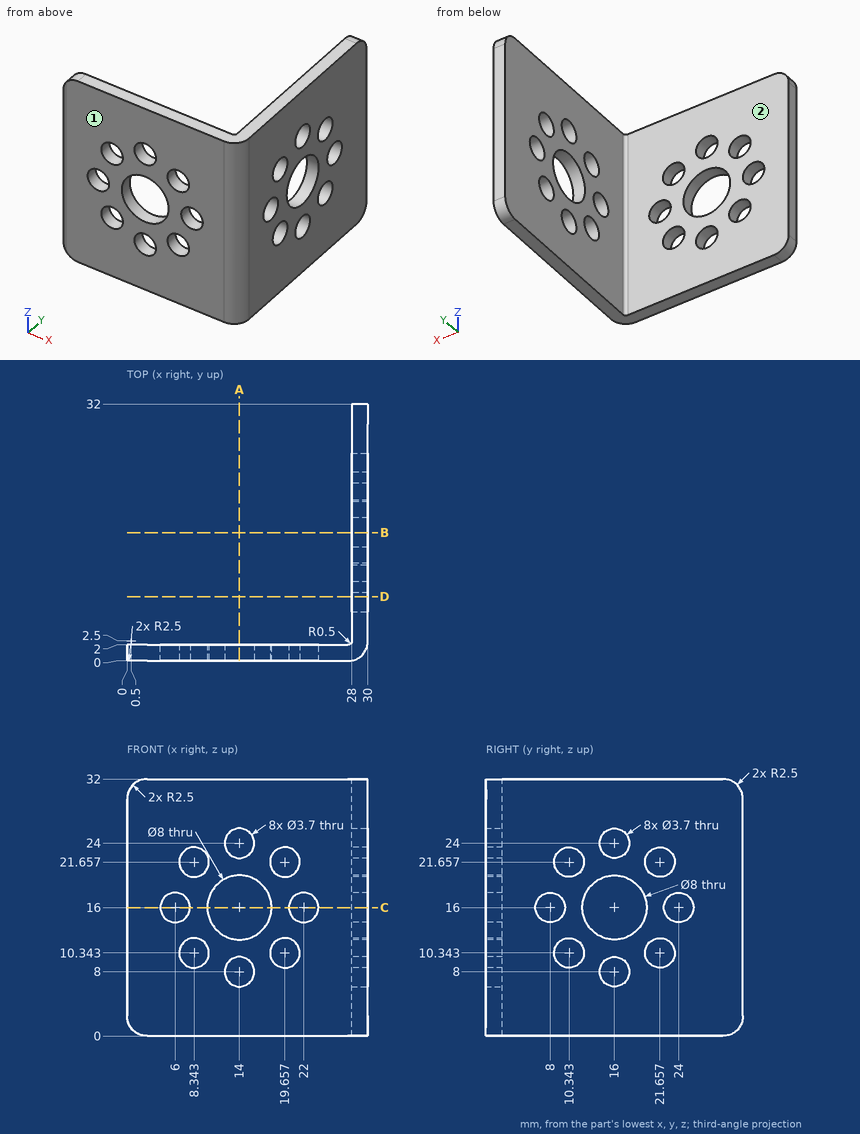
Answer from the drawing. Dimensions are ordinates in mm from the lowest x, y and z of the part. A direction names the side the tool comes from. Round coordinates to 2 decimals unless told otherwise and drop trailing zeros. Loops run counter-clockwise (first coordinate to the right, second up) from the corner with the lowest first, then second, coordinate; pieces in that order, holes last.
(1) The part is cut by section D-D, the plane y = 8. Give the vertices of the cut face in (x, z), and give its area (3 significant figures).
Computed values:
outline: (28, 0) - (30, 0) - (30, 14.15) - (28, 14.15) - close; (28, 17.85) - (30, 17.85) - (30, 32) - (28, 32) - close
area: 56.6 mm2
(2) Each of these flat-tipped pins is pushed along its axis until it touches: P1, Ø5, axis at x = 16, z = 13.5, coming from the -Y side; P2, Ø6, axis at x = 8.34, z = 21.66, coming from the +Y side; P3, Ø2, axis at y = 13, z = 22.5, coming from the -X side. Where does it stop, or does it pass through?
Computed values:
P1: stops at y = 0
P2: stops at y = 2
P3: stops at x = 28
(3) The part is cut by section C-C, the plane z = 16. Give the number of separate pieces and of enclosed holes in the cut face, and give its area (3 significant figures).
Computed values:
separate pieces: 7
enclosed holes: 0
area: 57.1 mm2
(4) For the marked faces 1 and 2, determine the directions among +Z, -Z, +X, -X, +Y, -Y from which every point of the face is accessible in a straight line to the end or side of a thin tool.
Computed values:
face 1: +Z, -Z, +X, -X, -Y
face 2: +Z, -Z, -X, +Y
(5) Find the intervals of material crossed by L1, parallel to Z at x = 29, y = 24; L2, parallel to Y at x = 29.5, z = 24; L3, parallel to Y at x = 17.5, z = 28.5, in increasing order.
Computed values:
L1: z = 0 to 14.15, 17.85 to 32
L2: y = 1 to 14.15, 17.85 to 32
L3: y = 0 to 2
(6) The part is cut by section B-B, the plane y = 16. Give the vertices of the cut face in (x, z).
Computed values:
outline: (28, 0) - (30, 0) - (30, 6.15) - (28, 6.15) - close; (28, 9.85) - (30, 9.85) - (30, 12) - (28, 12) - close; (28, 20) - (30, 20) - (30, 22.15) - (28, 22.15) - close; (28, 25.85) - (30, 25.85) - (30, 32) - (28, 32) - close
(7) The part is cut by section A-A, the plane x = 14. Give the vertices of the cut face in (y, z).
Computed values:
outline: (0, 0) - (2, 0) - (2, 6.15) - (0, 6.15) - close; (0, 9.85) - (2, 9.85) - (2, 12) - (0, 12) - close; (0, 20) - (2, 20) - (2, 22.15) - (0, 22.15) - close; (0, 25.85) - (2, 25.85) - (2, 32) - (0, 32) - close
